Design review of the part built by this model. Coordinates are the model's own, in mm. Face numbers are marked on the shaded views. A direction names the side the tool comes from. Give positions to 0.01 mm unless a question says otherwise; leave off trailing zeros. Loops run counter-clockwise (first coordinate to the right, second up) from the corner with the lowest first, then second, coordinate; pieces in that order, holes last. Notation, with made-up numbers: (76, 13) - (117, 13) arc R11 cw to (117, 17) - close; hole circle Ø1 at (20.25, 59.5). An arc over 180 degrees is marked (long way). Write each question's results on one line, items separated by ' | '.
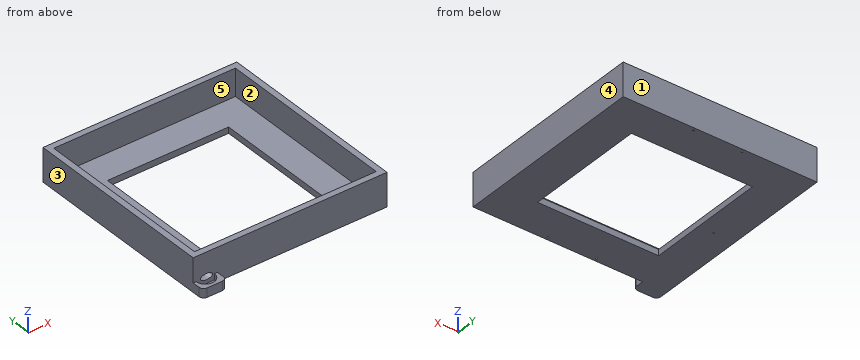
from build123d import *

# Parameters (mm, degrees)
F0_W      = 320
F0_H      = 320
F1_DEPTH  = 10
F2_W      = 320
F2_H      = 320
F2_W_2    = 300
F2_H_2    = 300
F3_DEPTH  = 45
F4_W      = 200
F4_H      = 200
F5_DEPTH  = 25
F6_W      = 40
F6_H      = 15
F7_DEPTH  = 20
F9_DEPTH  = 10
F10_R     = 7.5
F12_DEPTH = 10
F13_R     = 1.5
F14_DEPTH = 25
F15_R     = 1
F16_DEPTH = 5


with BuildPart() as f1:
    # F0 (on Top) → F1 (new body)
    with BuildSketch(Plane.XY):
        Rectangle(F0_W, F0_H)
    extrude(amount=F1_DEPTH)

    # F2 (on face) → F3 (join)
    with BuildSketch(Plane.XY.offset(10)):
        Rectangle(F2_W, F2_H)
        Rectangle(F2_W_2, F2_H_2, mode=Mode.SUBTRACT)
    extrude(amount=F3_DEPTH)

    # F4 (on face) → F5 (cut)
    with BuildSketch(Plane.XY.offset(10)):
        Rectangle(F4_W, F4_H)
    extrude(amount=-F5_DEPTH, mode=Mode.SUBTRACT)

    # F6 (on face) → F7 (join)
    with BuildSketch(Plane.XZ.offset(160)):
        with Locations((-140, 7.5)):
            Rectangle(F6_W, F6_H)
    extrude(amount=F7_DEPTH)

    # F8 (on face) → F9 (cut)
    with BuildSketch(Plane.XY.offset(15)):
        with BuildLine():
            Line((-125, -160), (-155, -160))
            ThreePointArc((-155, -160), (-140, -175), (-125, -160))
        make_face()
    extrude(amount=-F9_DEPTH, mode=Mode.SUBTRACT)

    # F10
    f10_edges = [f1.edges().sort_by_distance(p)[0] for p in [
        (-120, -180, 7.5),
        (-160, -180, 7.5),
    ]]
    fillet(f10_edges, radius=F10_R)

    # F11 (on face) → F12 (cut)
    with BuildSketch(Plane(origin=(0, -150, 0), x_dir=(-1, 0, 0), z_dir=(0, 1, 0))):
        with BuildLine():
            add(Edge.make_bspline(
                [(138, 11), (148, 11), (148, 16)],
                knots=[4.7123889804, 4.7123889804, 4.7123889804, 6.2831853072, 6.2831853072, 6.2831853072], degree=2, weights=[1, 0.7071067812, 1]))
            add(Edge.make_bspline(
                [(148, 16), (148, 28.0710678119), (130.9289321881, 19.5355339059), (113.8578643763, 11), (138, 11)],
                knots=[0, 0, 0, 2.3561944902, 2.3561944902, 4.7123889804, 4.7123889804, 4.7123889804], degree=2, weights=[1, 0.3826834324, 1, 0.3826834324, 1]))
        make_face()
    extrude(amount=-F12_DEPTH, mode=Mode.SUBTRACT)

    # F13 (on face) → F14 (cut)
    with BuildSketch(Plane(origin=(0, 0, 0), x_dir=(1, 0, 0), z_dir=(0, 0, -1))):
        with Locations((-40, 155)):
            Circle(F13_R)
        with Locations((40, 155)):
            Circle(F13_R)
        with Locations((40, -155)):
            Circle(F13_R)
        with Locations((-40, -155)):
            Circle(F13_R)
    extrude(amount=-F14_DEPTH, mode=Mode.SUBTRACT)

    # F15 (on face) → F16 (cut)
    with BuildSketch(Plane(origin=(0, 0, 0), x_dir=(1, 0, 0), z_dir=(0, 0, -1))):
        with Locations((-125, 15)):
            Circle(F15_R)
    extrude(amount=-F16_DEPTH, mode=Mode.SUBTRACT)


solid = f1.part
(1) Insertion check: P1, Ø1.5, axis at x = -40, y = 155, coming from the -Z side; P2, Ø3, axis at x = -106.5, y = -111, coming from the -Z side; P3, Ø4, axis at y = -163.5, z = 7.5, coming from the +X side; P4, Ø2.5, axis at x = -125, y = -15, coming from the +Z side. Each pin has a flat end and moves straight along its axis. Give the tip position at first contact, or say it passes through.
Answers below:
P1: z = 25 | P2: z = 0 | P3: x = -120 | P4: z = 10
(2) Take a section at C-C on z = 34. Give the boundary of the cut face in (x, y).
Answers below:
outline: (-160, -160) - (160, -160) - (160, 160) - (-160, 160) - close; hole (-150, -150) - (150, -150) - (150, 150) - (-150, 150) - close
(3) Tool access review of the marked faces 1 and 2: name each direction out of +Z, -Z, +X, -X, +Y, -Y from which nothing blocks a thin tool from reaching the whole face with its end or side.
Answers below:
face 1: +Z, -Z, +X, -X, +Y | face 2: +Z
(4) Wall thickness on line 1 along X through (y, z) = (-155, 6); line 2 along X through (y, z) = (-15, 2.8); line 3 along Y through (x, z) = (40, 19.75): over which ranges is each line inside the solid? List them lowest first. Write a range as from..to.
Answers below:
line 1: -160..-41.5, -38.5..38.5, 41.5..160 | line 2: -160..-126, -124..-100, 100..160 | line 3: -160..-156.5, -153.5..-150, 150..153.5, 156.5..160
(5) Take a section at D-D on y = 115. Give the boundary of the cut face in (x, z), plus the area to 3 significant figures.
Answers below:
outline: (-160, 0) - (160, 0) - (160, 55) - (150, 55) - (150, 10) - (-150, 10) - (-150, 55) - (-160, 55) - close | area: 4,100 mm2
(6) Take a section at A-A on y = -31.5. Give the boundary of the cut face in (x, z).
Answers below:
outline: (-160, 0) - (-100, 0) - (-100, 10) - (-150, 10) - (-150, 55) - (-160, 55) - close; (100, 0) - (160, 0) - (160, 55) - (150, 55) - (150, 10) - (100, 10) - close
(7) Draft analysis for pull direction X (two halves, no side actions). For the marked faces 3, 4 and 5, state which applies: pulls with the +X half, pulls with the -X half, needs draft (parallel to the pull), parting line crosses it, or undercut.
Answers below:
face 3: pulls with the -X half | face 4: pulls with the +X half | face 5: undercut
